Work out the finished part from the listing and answer in its coordinate system (mm). Face numbers are marked on the shaded views. A direction names the side the tool comes from. Coordinates: 2 decimals unless noted, no trailing zeros. Write each loop counter-clockwise with the first axis right and the second up, starting at its lowest first coordinate (ties: lowest second). Pieces come first, ordered by that corner, then holes. Notation, with made-up numbers: M 10,48 L 59,48 A28 ccw 59,77 Z; hole C 6,31 d10. An arc over 180 degrees is marked long. Answer as CSV lines item,"result". Start each with the question number.
(1) Find the intervals of material crossed by L1, parallel to X at y = 8.5, z = 10.5; L2, parallel to Y at x = 9.75, z = -1; L3, parallel to Y at x = 6.25, z = 12, in increasing order. Write a range as [from, to].
(2) For the marked faces 4, 5 and 6, determine the directions among +Z, -Z, +X, -X, +Y, -Y from which every point of the face is accessible in a straight line to the end or side of a thin tool.
(3) A cutting plane is placed at B-B on z = -7. Give the vertices of the cut face in (x, y).
(4) Flat-ended cylindrical pins translate along their axes: P1, Ø5, axis at x = 8.5, y = 18.5, coming from the +Z side; P2, Ø1.6, axis at x = -9.5, y = 23.5, coming from the -Z side; P3, Ø2.5, axis at x = 9.5, y = 23.5, coming from the +Z side; P4, Ø8, axis at x = 2, y = 14.5, coming from the -Z side. Find the tip coordinate at first contact, or state that the pin passes through.
(5) A cutting plane is placed at C-C on y = 12. Give the vertices of the cut face in (x, z).
(6) The mould has two halves that part along X. Classify the marked faces 1, 2 and 3: released by +X, released by -X, zero draft, split by the parting line, or undercut.
(7) A cutting plane is placed at D-D on y = -8. Give the vertices of the cut face in (x, z), then the cut area to 3 significant figures.
(8) A cutting plane is placed at A-A on z = 1.5. Give the vertices of the cut face in (x, y) (3 decimals).
from build123d import *

# Parameters (mm, degrees)
BOSS_EXTRUDE1_DEPTH = 11
SKETCH2_R           = 1
CUT_EXTRUDE1_DEPTH  = 37.813720268
CUT_EXTRUDE2_DEPTH  = 4.3
SKETCH6_R           = 8.5
BOSS_EXTRUDE2_DEPTH = 7
BOSS_EXTRUDE3_DEPTH = 5.9
CUT_EXTRUDE3_DEPTH  = 4
SKETCH9_R           = 0.3
BOSS_EXTRUDE4_DEPTH = 3.5
CUT_EXTRUDE4_START  = -6.34
CUT_EXTRUDE4_DEPTH  = 6.34
CUT_EXTRUDE5_START  = -6.96
CUT_EXTRUDE5_DEPTH  = 6.96
SKETCH14_R          = 0.8
CUT_EXTRUDE6_DEPTH  = 2
SKETCH15_R          = 1
CUT_EXTRUDE7_DEPTH  = 2
SKETCH16_R          = 3.575
CUT_EXTRUDE8_DEPTH  = 3
CUT_EXTRUDE9_START  = -0.7
CUT_EXTRUDE9_DEPTH  = 0.7
BOSS_EXTRUDE5_DEPTH = 2
SKETCH19_R          = 0.75
BOSS_EXTRUDE6_DEPTH = 5
BOSS_EXTRUDE7_DEPTH = 2.7
SKETCH21_R          = 0.8
CUT_EXTRUDE10_DEPTH = 1
BOSS_EXTRUDE8_START = 3
SKETCH22_R          = 5.6
SKETCH22_R_2        = 3.575
BOSS_EXTRUDE8_DEPTH = 3


with BuildPart() as part:
    # Sketch1 → Boss-Extrude1 (new, symmetric)
    with BuildSketch(Plane.XY):
        with BuildLine():
            Line((-7, 26.5), (7, 26.5))
            ThreePointArc((7, 26.5), (11.242640687, 24.742640687), (13, 20.5))
            Line((13, 20.5), (13, -20.5))
            Line((13, -20.5), (5.71, -20.5))
            Line((5.71, -20.5), (5.71, -22))
            Line((5.71, -22), (-5.71, -22))
            Line((-5.71, -22), (-5.71, -20.5))
            Line((-5.71, -20.5), (-13, -20.5))
            Line((-13, -20.5), (-13, 20.5))
            ThreePointArc((-13, 20.5), (-11.242640687, 24.742640687), (-7, 26.5))
        make_face()
    extrude(amount=BOSS_EXTRUDE1_DEPTH, both=True)

    # Sketch2 → Cut-Extrude1 (cut, through all)
    with BuildSketch(Plane.XY.offset(11)):
        with Locations((-9.5, 23.5)):
            Circle(SKETCH2_R)
        with Locations((-10.5, -18)):
            Circle(SKETCH2_R)
        with Locations((10.5, -18)):
            Circle(SKETCH2_R)
        with Locations((9.5, 23.5)):
            Circle(SKETCH2_R)
    extrude(amount=-CUT_EXTRUDE1_DEPTH, mode=Mode.SUBTRACT)

    # Sketch4 → Cut-Extrude2 (cut)
    with BuildSketch(Plane.XY.offset(11)):
        with BuildLine():
            Line((4.41, -19.2), (8.537858313, -19.2))
            ThreePointArc((8.537858313, -19.2), (8.873654403, -16.373654403), (11.7, -16.037858313))
            Line((11.7, -16.037858313), (11.7, 20.5))
            ThreePointArc((11.7, 20.5), (11.621181185, 21.357137361), (11.387368317, 22.185526403))
            ThreePointArc((11.387368317, 22.185526403), (8.027575881, 21.733091057), (7.866730044, 25.11939163))
            ThreePointArc((7.866730044, 25.11939163), (7.435235189, 25.179804518), (7, 25.2))
            Line((7, 25.2), (-7, 25.2))
            ThreePointArc((-7, 25.2), (-7.435235189, 25.179804518), (-7.866730044, 25.11939163))
            ThreePointArc((-7.866730044, 25.11939163), (-8.027575881, 21.733091057), (-11.387368317, 22.185526403))
            ThreePointArc((-11.387368317, 22.185526403), (-11.621181185, 21.357137361), (-11.7, 20.5))
            Line((-11.7, 20.5), (-11.7, -16.037858313))
            ThreePointArc((-11.7, -16.037858313), (-8.873654403, -16.373654403), (-8.537858313, -19.2))
            Line((-8.537858313, -19.2), (-4.41, -19.2))
            Line((-4.41, -19.2), (-4.41, -20.7))
            Line((-4.41, -20.7), (4.41, -20.7))
            Line((4.41, -20.7), (4.41, -19.2))
        make_face()
    extrude(amount=-CUT_EXTRUDE2_DEPTH, mode=Mode.SUBTRACT)

    # Sketch6 → Boss-Extrude2 (add)
    with BuildSketch(Plane.XY.offset(6.7)):
        with Locations(Location((0, -12.1, 0), (0, 0, 236.646476163))):
            Circle(SKETCH6_R)
    extrude(amount=BOSS_EXTRUDE2_DEPTH)

    # Sketch7 → Boss-Extrude3 (add)
    with BuildSketch(Plane.XY.offset(6.7)):
        Polygon((-1.5, -2.6), (0, -1.1), (0, -2.6), (8.4, -2.6), (9.9, -1.1), (9.9, 2.3), (-9.9, 2.3), (-9.9, -2.6), align=None)
    extrude(amount=BOSS_EXTRUDE3_DEPTH)

    # Sketch8 → Cut-Extrude3 (cut)
    with BuildSketch(Plane.XY.offset(12.6)):
        Polygon((-9.2, 1.6), (-9.2, -0.810050506), (-8.110050506, -1.9), (-6.789949494, -1.9), (-6.2, -1.310050506), (-5.610050506, -1.9), (-4.289949494, -1.9), (-3.7, -1.310050506), (-3.110050506, -1.9), (-1.789949494, -1.9), (-0.7, -0.810050506), (-0.7, 1.6), align=None)
        Polygon((5.610050506, -1.9), (4.289949494, -1.9), (3.7, -1.310050506), (3.110050506, -1.9), (1.789949494, -1.9), (0.7, -0.810050506), (0.7, 1.6), (9.2, 1.6), (9.2, -0.810050506), (8.110050506, -1.9), (6.789949494, -1.9), (6.2, -1.310050506), align=None)
    extrude(amount=-CUT_EXTRUDE3_DEPTH, mode=Mode.SUBTRACT)

    # Sketch9 → Boss-Extrude4 (add)
    with BuildSketch(Plane.XY.offset(8.6)):
        with Locations((-7.45, -0.78)):
            Circle(SKETCH9_R)
        with Locations((-4.95, -0.78)):
            Circle(SKETCH9_R)
        with Locations((-2.45, -0.78)):
            Circle(SKETCH9_R)
        with Locations(Location((2.45, -0.78, 0), (0, 0, 180))):
            Circle(SKETCH9_R)
        with Locations(Location((4.95, -0.78, 0), (0, 0, 180))):
            Circle(SKETCH9_R)
        with Locations(Location((7.45, -0.78, 0), (0, 0, 180))):
            Circle(SKETCH9_R)
    extrude(amount=BOSS_EXTRUDE4_DEPTH)

    # Sketch11 → Cut-Extrude4 (cut)
    with BuildSketch(Plane(origin=(0, 0, -11), x_dir=(-1, 0, 0), z_dir=(0, 0, -1)).offset(CUT_EXTRUDE4_START)):
        with BuildLine():
            Line((3.3, -3), (11.7, -3))
            Line((11.7, -3), (11.7, 20.5))
            ThreePointArc((11.7, 20.5), (11.621181185, 21.357137361), (11.387368317, 22.185526403))
            ThreePointArc((11.387368317, 22.185526403), (8.027575881, 21.733091057), (7.866730044, 25.11939163))
            ThreePointArc((7.866730044, 25.11939163), (7.435235189, 25.179804518), (7, 25.2))
            Line((7, 25.2), (-7, 25.2))
            ThreePointArc((-7, 25.2), (-7.435235189, 25.179804518), (-7.866730044, 25.11939163))
            ThreePointArc((-7.866730044, 25.11939163), (-8.027575881, 21.733091057), (-11.387368317, 22.185526403))
            ThreePointArc((-11.387368317, 22.185526403), (-11.621181185, 21.357137361), (-11.7, 20.5))
            Line((-11.7, 20.5), (-11.7, -5))
            Line((-11.7, -5), (-5, -5))
            ThreePointArc((-5, -5), (-1.958040085, -4.304480936), (0.479422369, -2.356137108))
            ThreePointArc((0.479422369, -2.356137108), (1.853433583, -2.836990264), (3.3, -3))
        make_face()
    extrude(amount=CUT_EXTRUDE4_DEPTH, mode=Mode.SUBTRACT)

    # Sketch12 → Cut-Extrude5 (cut)
    with BuildSketch(Plane(origin=(0, 0, -4.66), x_dir=(-1, 0, 0), z_dir=(0, 0, -1)).offset(CUT_EXTRUDE5_START)):
        with BuildLine():
            Line((7, 25.2), (-7, 25.2))
            ThreePointArc((-7, 25.2), (-7.435235189, 25.179804518), (-7.866730044, 25.11939163))
            ThreePointArc((-7.866730044, 25.11939163), (-8.027575881, 21.733091057), (-11.387368317, 22.185526403))
            ThreePointArc((-11.387368317, 22.185526403), (-11.621181185, 21.357137361), (-11.7, 20.5))
            Line((-11.7, 20.5), (-11.7, 15))
            ThreePointArc((-11.7, 15), (-9.334774926, 7.94649186), (-3.195388533, 3.744801551))
            ThreePointArc((-3.195388533, 3.744801551), (-1.381944579, -1.008813032), (3.3, -3))
            Line((3.3, -3), (11.7, -3))
            Line((11.7, -3), (11.7, 20.5))
            ThreePointArc((11.7, 20.5), (11.621181185, 21.357137361), (11.387368317, 22.185526403))
            ThreePointArc((11.387368317, 22.185526403), (8.027575881, 21.733091057), (7.866730044, 25.11939163))
            ThreePointArc((7.866730044, 25.11939163), (7.435235189, 25.179804518), (7, 25.2))
        make_face()
    extrude(amount=CUT_EXTRUDE5_DEPTH, mode=Mode.SUBTRACT)

    # Sketch14 → Cut-Extrude6 (cut)
    with BuildSketch(Plane(origin=(0, 0, -4.66), x_dir=(-1, 0, 0), z_dir=(0, 0, -1))):
        with Locations((-5, 2)):
            Circle(SKETCH14_R)
    extrude(amount=-CUT_EXTRUDE6_DEPTH, mode=Mode.SUBTRACT)

    # Sketch15 → Cut-Extrude7 (cut)
    with BuildSketch(Plane(origin=(0, 0, 2.3), x_dir=(-1, 0, 0), z_dir=(0, 0, -1))):
        with Locations((3.3, 3.5)):
            Circle(SKETCH15_R)
    extrude(amount=-CUT_EXTRUDE7_DEPTH, mode=Mode.SUBTRACT)

    # Sketch16 → Cut-Extrude8 (cut)
    with BuildSketch(Plane(origin=(0, 0, 2.3), x_dir=(-1, 0, 0), z_dir=(0, 0, -1))):
        with Locations((0, 15)):
            Circle(SKETCH16_R)
    extrude(amount=-CUT_EXTRUDE8_DEPTH, mode=Mode.SUBTRACT)

    # Sketch17 → Cut-Extrude9 (cut)
    with BuildSketch(Plane(origin=(0, 0, -11), x_dir=(-1, 0, 0), z_dir=(0, 0, -1)).offset(CUT_EXTRUDE9_START)):
        with BuildLine():
            Line((4.41, -20.7), (4.41, -19.2))
            Line((4.41, -19.2), (8.537858313, -19.2))
            ThreePointArc((8.537858313, -19.2), (8.873654403, -16.373654403), (11.7, -16.037858313))
            Line((11.7, -16.037858313), (11.7, 20.5))
            ThreePointArc((11.7, 20.5), (11.621181185, 21.357137361), (11.387368317, 22.185526403))
            ThreePointArc((11.387368317, 22.185526403), (8.027575881, 21.733091057), (7.866730044, 25.11939163))
            ThreePointArc((7.866730044, 25.11939163), (7.435235189, 25.179804518), (7, 25.2))
            Line((7, 25.2), (-7, 25.2))
            ThreePointArc((-7, 25.2), (-7.435235189, 25.179804518), (-7.866730044, 25.11939163))
            ThreePointArc((-7.866730044, 25.11939163), (-8.027575881, 21.733091057), (-11.387368317, 22.185526403))
            ThreePointArc((-11.387368317, 22.185526403), (-11.621181185, 21.357137361), (-11.7, 20.5))
            Line((-11.7, 20.5), (-11.7, -16.037858313))
            ThreePointArc((-11.7, -16.037858313), (-8.873654403, -16.373654403), (-8.537858313, -19.2))
            Line((-8.537858313, -19.2), (-4.41, -19.2))
            Line((-4.41, -19.2), (-4.41, -20.7))
            Line((-4.41, -20.7), (4.41, -20.7))
        make_face()
    extrude(amount=CUT_EXTRUDE9_DEPTH, mode=Mode.SUBTRACT)

    # Sketch18 → Boss-Extrude5 (add)
    with BuildSketch(Plane(origin=(0, 0, -10.3), x_dir=(-1, 0, 0), z_dir=(0, 0, -1))):
        with BuildLine():
            Line((-4.462062303, -20.6), (4.462062303, -20.6))
            ThreePointArc((4.462062303, -20.6), (9.568945301, -11.328452318), (3.042556406, -2.994899753))
            ThreePointArc((3.042556406, -2.994899753), (1.728199092, -2.807094569), (0.479422369, -2.356137108))
            ThreePointArc((0.479422369, -2.356137108), (-1.958040085, -4.304480936), (-5, -5))
            Line((-5, -5), (-6.461423992, -5))
            ThreePointArc((-6.461423992, -5), (-9.522113117, -13.320394113), (-4.462062303, -20.6))
        make_face()
    extrude(amount=BOSS_EXTRUDE5_DEPTH)

    # Sketch19 → Boss-Extrude6 (add)
    with BuildSketch(Plane(origin=(0, 0, -12.3), x_dir=(-1, 0, 0), z_dir=(0, 0, -1))):
        with Locations((0, -12.1)):
            Circle(SKETCH19_R)
    extrude(amount=BOSS_EXTRUDE6_DEPTH)

    # Sketch20 → Boss-Extrude7 (add)
    with BuildSketch(Plane(origin=(0, 0, -17.3), x_dir=(-1, 0, 0), z_dir=(0, 0, -1))):
        Polygon((-0.352165696, -10.900633783), (0, -10.475), (0.352165696, -10.900633783), (0.878541328, -10.732963009), (0.944686968, -11.281424083), (1.478151992, -11.424950604), (1.237276802, -11.922106452), (1.608459843, -12.331261612), (1.137039994, -12.619268766), (1.228093058, -13.164148693), (0.675801022, -13.151566916), (0.457815405, -13.659176082), (0, -13.35), (-0.457815405, -13.659176082), (-0.675801022, -13.151566916), (-1.228093058, -13.164148693), (-1.137039994, -12.619268766), (-1.608459843, -12.331261612), (-1.237276802, -11.922106452), (-1.478151992, -11.424950604), (-0.944686968, -11.281424083), (-0.878541328, -10.732963009), align=None)
    extrude(amount=-BOSS_EXTRUDE7_DEPTH)

    # Sketch21 → Cut-Extrude10 (cut)
    with BuildSketch(Plane(origin=(0, 0, -12.3), x_dir=(-1, 0, 0), z_dir=(0, 0, -1))):
        with Locations((0.8, -4.7)):
            Circle(SKETCH21_R)
    extrude(amount=-CUT_EXTRUDE10_DEPTH, mode=Mode.SUBTRACT)

    # Sketch22 → Boss-Extrude8 (add)
    with BuildSketch(Plane(origin=(0, 0, 2.3), x_dir=(-1, 0, 0), z_dir=(0, 0, -1)).offset(BOSS_EXTRUDE8_START)):
        with Locations(Location((0, 15, 0), (0, 0, 180))):
            Circle(SKETCH22_R)
        with Locations((0, 15)):
            Circle(SKETCH22_R_2, mode=Mode.SUBTRACT)
    extrude(amount=-BOSS_EXTRUDE8_DEPTH)


solid = part.part
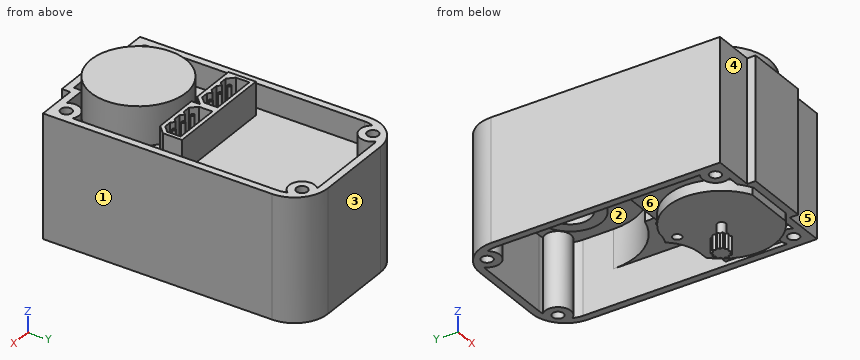
Here are the results:
1,L1,"x = [-13, -11.7], [11.7, 13]"
1,L2,"y = [-20.5, -18.66], [-17.34, 8.53], [21.21, 22.53], [24.47, 25.83]"
1,L3,"y = [-17.86, -6.34], [-2.6, -1.36], [1.6, 2.3]"
2,face 4,"+Z, -Z, -X, -Y"
2,face 5,"+Z, -Z, +X, -Y"
2,face 6,"-Z"
3,outline,"M -13,-20.5 L -5.71,-20.5 L -5.71,-22 L 5.71,-22 L 5.71,-20.5 L 13,-20.5 L 13,20.5 A6 ccw 7,26.5 L -7,26.5 A6 ccw -13,20.5 Z; hole M -11.7,-3 L -3.3,-3 A6.5 ccw -0.48,-2.36 A7 ccw 5,-5 L 11.7,-5 L 11.7,20.5 A4.7 ccw 11.39,22.19 A2.3 cw long 7.87,25.12 A4.7 ccw 7,25.2 L -7,25.2 A4.7 ccw -7.87,25.12 A2.3 cw long -11.39,22.19 A4.7 ccw -11.7,20.5 Z; hole C -10.5,-18 d2; hole C -9.5,23.5 d2; hole C 9.5,23.5 d2; hole C 10.5,-18 d2"
4,P1,"stops at z = 6.7"
4,P2,"passes through"
4,P3,"stops at z = 11"
4,P4,"stops at z = -0.7"
5,outline,"M -13,-11 L -11.7,-11 L -11.7,2.3 L -4.73,2.3 L -4.73,-0.7 L -1.94,-0.7 L -1.94,5.3 L 1.94,5.3 L 1.94,-0.7 L 4.73,-0.7 L 4.73,2.3 L 11.31,2.3 L 11.31,-4.66 L 11.7,-4.66 L 11.7,-11 L 13,-11 L 13,11 L 11.7,11 L 11.7,6.7 L -11.7,6.7 L -11.7,11 L -13,11 Z"
6,face 1,"released by +X"
6,face 2,"undercut"
6,face 3,"zero draft"
7,outline,"M -13,-11 L -11.7,-11 L -11.7,-10.3 L -8.68,-10.3 L -8.68,-12.3 L 8.68,-12.3 L 8.68,-10.3 L 11.7,-10.3 L 11.7,-11 L 13,-11 L 13,11 L 11.7,11 L 11.7,6.7 L 7.45,6.7 L 7.45,13.7 L -7.45,13.7 L -7.45,6.7 L -11.7,6.7 L -11.7,11 L -13,11 Z"
7,area,"594 mm^2"
8,outline,"M -13,-20.5 L -5.71,-20.5 L -5.71,-22 L 5.71,-22 L 5.71,-20.5 L 13,-20.5 L 13,20.5 A6 ccw 7,26.5 L -7,26.5 A6 ccw -13,20.5 Z; C 0,15 d11.2; hole M -11.7,-3 L -3.3,-3 A6.5 ccw 3.195,3.745 A11.7 ccw 11.7,15 L 11.7,20.5 A4.7 ccw 11.387,22.186 A2.3 cw long 7.867,25.119 A4.7 ccw 7,25.2 L -7,25.2 A4.7 ccw -7.867,25.119 A2.3 cw long -11.387,22.186 A4.7 ccw -11.7,20.5 Z; hole C -10.5,-18 d2; hole C -9.5,23.5 d2; hole C 0,15 d7.15; hole C 9.5,23.5 d2; hole C 10.5,-18 d2"
